Could you check a few things on this model? Use its own coordinates, in mm. Face numbers are marked on the shaded views. A direction names the side the tool comes from. Give positions to 0.01 mm unless a question says otherwise; leave off trailing zeros. Loops run counter-clockwise (first coordinate to the right, second up) from the corner with the lowest first, then second, coordinate; pieces in that order, holes last. Notation, with made-up numbers: (-11.5, -38.5) - (43.5, -38.5) arc R25 ccw to (43.5, -22.5) - close; hole circle Ø11 at (-36.5, 14.25). An arc over 180 degrees is marked (long way). One line per item, written item: value. Start each with the question number.
Q1. For the marked faces 1, 2, 3, 4 and 5, which set-ups out of +Z, -Z, +X, -X, +Y, -Y let a thin tool reach every point of the face, with its end or its side?
Q2. I'm going to push flat-ended pins straight in: P1, Ø2, axis at y = -19.5, z = 6, coming from the -X side; P2, Ø4, axis at x = -35.2, y = 26.4, coming from the +Z side; P3, Ø3, axis at x = -35.2, y = -26.4, coming from the +Z side; P4, Ø5, axis at y = -9, z = 4, coming from the -X side. Where does each tip first touch, or does it pass through?
Q3. I want a section at C-C (z = -22). Please give me the cut outline in (x, y).
Q4. If I drill on line 1 (Y direction, x = -35.2, z = -3); line 2 (Y direction, x = -6.5, z = 2.5); line 3 (X direction, y = -26, z = -1) (3 decimals), over which ranges is the centre line in solid material (lowest first)? Write a range as from..to.
Q5. I want a section at B-B (y = 22). Please give me the cut outline in (x, z).
Q6. If we mould it in two halves opening along Y, with no side actions, what happens to the marked faces 6, 7 and 8? For each: released by +Y, released by -Y, zero draft, split by the parting line, or undercut.
Q7. I want a section at A-A (x = 17). Please give me the cut outline in (y, z).
```python
from build123d import *

# Parameters (mm, degrees)
BOSS_EXTRUDE3_DEPTH = 12
CUT_EXTRUDE1_DEPTH  = 12
SKETCH7_W           = 80
SKETCH7_H           = 60
BOSS_EXTRUDE4_DEPTH = 5
BOSS_EXTRUDE5_DEPTH = 30
SKETCH10_R          = 1.8
CUT_EXTRUDE2_DEPTH  = 30
CUT_EXTRUDE3_DEPTH  = 10


with BuildPart() as part:
    # Sketch5 → Boss-Extrude3 (new body)
    with BuildSketch(Plane.XY):
        with BuildLine():
            Line((10, -28), (-10, -28))
            ThreePointArc((-10, -28), (-38, 0), (-10, 28))
            Line((-10, 28), (10, 28))
            ThreePointArc((10, 28), (38, 0), (10, -28))
        make_face()
    extrude(amount=BOSS_EXTRUDE3_DEPTH)

    # Sketch6 → Cut-Extrude1 (cut)
    with BuildSketch(Plane.XY.offset(12)):
        with BuildLine():
            Line((10, -25), (-10, -25))
            ThreePointArc((-10, -25), (-35, 0), (-10, 25))
            Line((-10, 25), (10, 25))
            ThreePointArc((10, 25), (35, 0), (10, -25))
        make_face()
    extrude(amount=-CUT_EXTRUDE1_DEPTH, mode=Mode.SUBTRACT)

    # Sketch7 → Boss-Extrude4 (add)
    with BuildSketch(Plane(origin=(0, 0, 0), x_dir=(-1, 0, 0), z_dir=(0, 0, -1))):
        Rectangle(SKETCH7_W, SKETCH7_H)
        with BuildLine():
            Line((10, -25), (-10, -25))
            ThreePointArc((-10, -25), (-35, 0), (-10, 25))
            Line((-10, 25), (10, 25))
            ThreePointArc((10, 25), (35, 0), (10, -25))
        make_face(mode=Mode.SUBTRACT)
    extrude(amount=BOSS_EXTRUDE4_DEPTH)

    # Sketch9 → Boss-Extrude5 (add)
    with BuildSketch(Plane(origin=(0, 0, -5), x_dir=(-1, 0, 0), z_dir=(0, 0, -1))):
        with BuildLine():
            Line((10, -28), (-10, -28))
            ThreePointArc((-10, -28), (-38, 0), (-10, 28))
            Line((-10, 28), (10, 28))
            ThreePointArc((10, 28), (38, 0), (10, -28))
        make_face()
        with BuildLine():
            Line((10, -25), (-10, -25))
            ThreePointArc((-10, -25), (-35, 0), (-10, 25))
            Line((-10, 25), (10, 25))
            ThreePointArc((10, 25), (35, 0), (10, -25))
        make_face(mode=Mode.SUBTRACT)
    extrude(amount=BOSS_EXTRUDE5_DEPTH)

    # Sketch10 → Cut-Extrude2 (cut)
    with BuildSketch(Plane(origin=(0, 0, -5), x_dir=(-1, 0, 0), z_dir=(0, 0, -1))):
        with Locations((-35.2, 26.4)):
            Circle(SKETCH10_R)
        with Locations((35.2, 26.4)):
            Circle(SKETCH10_R)
        with Locations((35.2, -26.4)):
            Circle(SKETCH10_R)
        with Locations((-35.2, -26.4)):
            Circle(SKETCH10_R)
    extrude(amount=-CUT_EXTRUDE2_DEPTH, mode=Mode.SUBTRACT)

    # Sketch11 → Cut-Extrude3 (cut)
    with BuildSketch(Plane(origin=(0, 0, -35), x_dir=(-1, 0, 0), z_dir=(0, 0, -1))):
        with BuildLine():
            Line((10, -26), (-10, -26))
            ThreePointArc((-10, -26), (-36, 0), (-10, 26))
            Line((-10, 26), (10, 26))
            ThreePointArc((10, 26), (36, 0), (10, -26))
        make_face()
    extrude(amount=-CUT_EXTRUDE3_DEPTH, mode=Mode.SUBTRACT)


solid = part.part
```
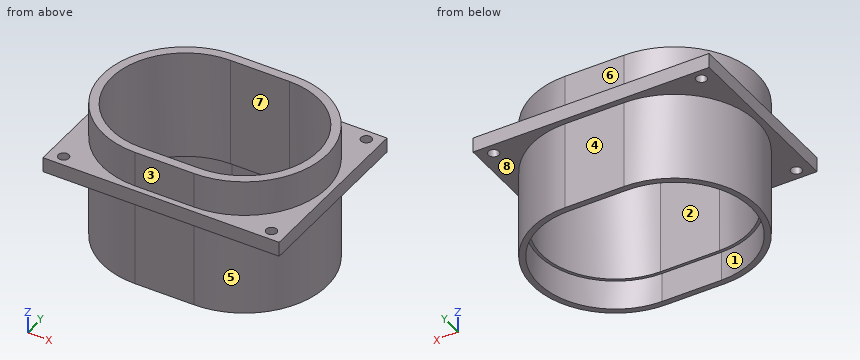
Worked answers:
1. face 1: -Z
1. face 2: +Z, -Z
1. face 3: +Z, +X, -X, -Y
1. face 4: -Z, +X, -X, +Y
1. face 5: -Z, +X
2. P1: stops at x = -31.02
2. P2: stops at z = 0
2. P3: passes through
2. P4: stops at x = -37.24
3. outline: (-10, -28) - (10, -28) arc R28 ccw to (10, 28) - (-10, 28) arc R28 ccw to start; hole (-10, -25) - (10, -25) arc R25 ccw to (10, 25) - (-10, 25) arc R25 ccw to start
4. line 1: y = -30..-28.2, -24.6..24.6, 28.2..30
4. line 2: y = -28..-25, 25..28
4. line 3: x = -40..-36.955, -33.445..33.445, 36.955..40
5. outline: (-40, -5) - (-27.32, -5) - (-27.32, -35) - (-23.86, -35) - (-23.86, -25) - (-21.87, -25) - (-21.87, 12) - (-27.32, 12) - (-27.32, 0) - (-40, 0) - close; (21.87, -25) - (23.86, -25) - (23.86, -35) - (27.32, -35) - (27.32, -5) - (40, -5) - (40, 0) - (27.32, 0) - (27.32, 12) - (21.87, 12) - close
6. face 6: released by +Y
6. face 7: undercut
6. face 8: zero draft
7. outline: (-30, -5) - (-27.11, -5) - (-27.11, -35) - (-25.04, -35) - (-25.04, -25) - (-24, -25) - (-24, 12) - (-27.11, 12) - (-27.11, 0) - (-30, 0) - close; (24, -25) - (25.04, -25) - (25.04, -35) - (27.11, -35) - (27.11, -5) - (30, -5) - (30, 0) - (27.11, 0) - (27.11, 12) - (24, 12) - close
